CAD build for the part. Positions are in the model's coordinates, mm. Coordinates: 2 decimals unless noted, no trailing zeros. Write each loop counter-clockwise with the first axis right and the second up, starting at its lowest first coordinate (ties: lowest second). Pieces come first, ordered by that corner, then holes. Notation, with made-up numbers: (-7.75, 35.5) - (37.25, 35.5) arc R20 ccw to (37.25, 51.5) - close; hole circle Ø11 at (2, 50). An arc over 180 degrees is marked (long way). One line per question, with ' | ' between items. Start each with the question number.
1. Flat gauge pins, fed straight in: P1, Ø3, axis at x = -3.5, y = 357, coming from the +Z side; P2, Ø2.5, axis at x = 0.5, z = 1, coming from the +Y side; P3, Ø5, axis at x = 4, y = 135, coming from the -Z side. Where does each tip first touch, or does it go through?
2. Band-saw the part on A-A, the plane z = 0. Write the cut outline in (x, y), then the cut area to 3 significant figures.
3. Probe line 1 (X direction, y = 6.5, z = 0); line 2 (Z direction, x = 0, y = 541); line 3 (X direction, y = 517, z = 5.25). List the from-to ranges inside material, lowest first.
4. Band-saw the part on B-B, the plane y = 331. Write the cut outline in (x, z), then the cut area to 3 significant figures.
Autodesk Inventor part; units mm, degrees
ref_plane "YZ Plane" through (0, 0, 0) normal (1, 0, 0) x (0, 1, 0)
ref_plane "XZ Plane" through (0, 0, 0) normal (0, 1, 0) x (-1, 0, 0)
ref_plane "XY Plane" through (0, 0, 0) normal (0, 0, 1) x (1, 0, 0)
sketch "Sketch1" plane through (0, 0, 0) normal (0, 1, 0) x (-1, 0, 0)
  line L0 (6.35, -3.6662) -> (0, -7.3323)
  line L1 (0, -7.3323) -> (-6.35, -3.6662)
  line L2 (-6.35, -3.6662) -> (-6.35, 3.6662)
  line L3 (-6.35, 3.6662) -> (0, 7.3323)
  line L4 (0, 7.3323) -> (6.35, 3.6662)
  line L5 (6.35, 3.6662) -> (6.35, -3.6662)
  point P0 (0, 0)
  point P1 (0, 0)
  point P2 (0, 0)
  dimension "d0" = 12.7
extrude "Extrusion1" add sketch "Sketch1" along normal blind 559.4858
sketch "Sketch2" plane through (0, 0, 0) normal (0, -1, 0) x (1, 0, 0)
  point P0 (0, 0)
  point P1 (0, 0)
hole "Hole1" at (0, 0, 0) direction (0, 1, 0) diameter 4.9784 depth 25.4
sketch "Sketch3" plane through (0, 559.4858, 0) normal (0, 1, 0) x (1, 0, 0)
  point P0 (0, 0)
  point P1 (0, 0)
hole "Hole2" at (0, 559.4858, 0) direction (0, -1, 0) diameter 4.9784 depth 25.4
properties part number "Intake Hex Shaft 3" material "Aluminum 6061"
Filled in:
1) P1: stops at z = 6.18 | P2: stops at y = 534.09 | P3: stops at z = -6.47
2) outline: (-6.35, 0) - (-2.49, 0) - (-2.49, 25.4) - (2.49, 25.4) - (2.49, 0) - (6.35, 0) - (6.35, 559.49) - (2.49, 559.49) - (2.49, 534.09) - (-2.49, 534.09) - (-2.49, 559.49) - (-6.35, 559.49) - close | area: 6,850 mm²
3) line 1: x = -6.35 to -2.49, 2.49 to 6.35 | line 2: z = -7.33 to -2.49, 2.49 to 7.33 | line 3: x = -3.61 to 3.61
4) outline: (-6.35, -3.67) - (0, -7.33) - (6.35, -3.67) - (6.35, 3.67) - (0, 7.33) - (-6.35, 3.67) - close | area: 140 mm²
